Can you work these out from the model? Positions are in its coordinate system, mm. Face numbers are marked on the shaded views. A direction names the side the tool comes from. Coordinates: 2 decimals unless noted, no trailing zeros. Loops run counter-clockwise (first coordinate to the right, second up) from the corner with the lowest first, then second, coordinate; pieces in that order, holes last.
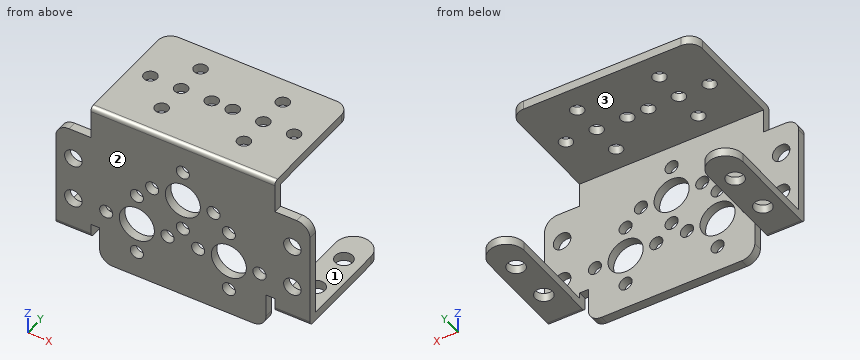
```python
from build123d import *

# Parameters (mm, degrees)
SKETCH1_R               = 2
SKETCH1_R_2             = 4
SKETCH1_R_3             = 1.5
BOSS_EXTRUDE1_DEPTH     = 27
SKETCH3_W               = 28.5
SKETCH3_H               = 26.527175283
SKETCH3_W_2             = 6.268481117
CUT_EXTRUDE1_DEPTH      = 30
CUT_EXTRUDE1_DEPTH_BACK = 30
SKETCH4_R               = 2
SKETCH4_R_2             = 1.5
CUT_EXTRUDE2_DEPTH      = 38.5
SKETCH5_W               = 38
SKETCH5_H               = 27.064125823
CUT_EXTRUDE3_DEPTH      = 27
FILLET1_R               = 3
FILLET2_R               = 1


with BuildPart() as part:
    # Sketch1 → Boss-Extrude1 (new body)
    with BuildSketch(Plane(origin=(0, 0, 0), x_dir=(1, 0, 0), z_dir=(0, 1, 0))):
        with BuildLine():
            Line((21, 0), (-21, 0))
            Line((-21, 0), (-21, 7.5))
            Line((-21, 7.5), (-26, 7.5))
            ThreePointArc((-26, 7.5), (-28.121320344, 8.378679656), (-29, 10.5))
            Line((-29, 10.5), (-29, 32.5))
            Line((-29, 32.5), (-21, 32.5))
            Line((-21, 32.5), (-21, 29.209337349))
            Line((-21, 29.209337349), (-19, 29.209337349))
            Line((-19, 29.209337349), (-19, 34.5))
            ThreePointArc((-19, 34.5), (-18.121320344, 36.621320344), (-16, 37.5))
            Line((-16, 37.5), (16, 37.5))
            ThreePointArc((16, 37.5), (18.121320344, 36.621320344), (19, 34.5))
            Line((19, 34.5), (19, 29.209337349))
            Line((19, 29.209337349), (21, 29.209337349))
            Line((21, 29.209337349), (21, 32.5))
            Line((21, 32.5), (29, 32.5))
            Line((29, 32.5), (29, 10.5))
            ThreePointArc((29, 10.5), (28.121320344, 8.378679656), (26, 7.5))
            Line((26, 7.5), (21, 7.5))
            Line((21, 7.5), (21, 0))
        make_face()
        with Locations((-25, 24.5)):
            Circle(SKETCH1_R, mode=Mode.SUBTRACT)
        with Locations((-25, 14.5)):
            Circle(SKETCH1_R, mode=Mode.SUBTRACT)
        with Locations((25, 14.5)):
            Circle(SKETCH1_R, mode=Mode.SUBTRACT)
        with Locations((25, 24.5)):
            Circle(SKETCH1_R, mode=Mode.SUBTRACT)
        with Locations((0, 14)):
            Circle(SKETCH1_R_2, mode=Mode.SUBTRACT)
        with Locations((0, 21)):
            Circle(SKETCH1_R_3, mode=Mode.SUBTRACT)
        with Locations((7, 14)):
            Circle(SKETCH1_R_3, mode=Mode.SUBTRACT)
        with Locations((0, 7)):
            Circle(SKETCH1_R_3, mode=Mode.SUBTRACT)
        with Locations((-7, 14)):
            Circle(SKETCH1_R_3, mode=Mode.SUBTRACT)
        with Locations((10.5, 24.5)):
            Circle(SKETCH1_R_2, mode=Mode.SUBTRACT)
        with Locations((10.5, 31.5)):
            Circle(SKETCH1_R_3, mode=Mode.SUBTRACT)
        with Locations((-10.5, 24.5)):
            Circle(SKETCH1_R_2, mode=Mode.SUBTRACT)
        with Locations((-10.5, 31.5)):
            Circle(SKETCH1_R_3, mode=Mode.SUBTRACT)
        with Locations((3.5, 24.5)):
            Circle(SKETCH1_R_3, mode=Mode.SUBTRACT)
        with Locations((10.5, 17.5)):
            Circle(SKETCH1_R_3, mode=Mode.SUBTRACT)
        with Locations((17.5, 24.5)):
            Circle(SKETCH1_R_3, mode=Mode.SUBTRACT)
        with Locations((-3.5, 24.5)):
            Circle(SKETCH1_R_3, mode=Mode.SUBTRACT)
        with Locations((-10.5, 17.5)):
            Circle(SKETCH1_R_3, mode=Mode.SUBTRACT)
        with Locations((-17.5, 24.5)):
            Circle(SKETCH1_R_3, mode=Mode.SUBTRACT)
    extrude(amount=BOSS_EXTRUDE1_DEPTH)

    # Sketch3 → Cut-Extrude1 (cut, two sides)
    with BuildSketch(Plane(origin=(0, 0, 0), x_dir=(0, 0, -1), z_dir=(1, 0, 0))) as cut_extrude1_sk:
        with Locations((16.25, 15.263587642)):
            Rectangle(SKETCH3_W, SKETCH3_H)
        with Locations((35.691254192, 15.263587642)):
            Rectangle(SKETCH3_W_2, SKETCH3_H)
    extrude(amount=CUT_EXTRUDE1_DEPTH, mode=Mode.SUBTRACT)
    extrude(cut_extrude1_sk.sketch, amount=-CUT_EXTRUDE1_DEPTH_BACK, mode=Mode.SUBTRACT)

    # Sketch4 → Cut-Extrude2 (cut, through all)
    with BuildSketch(Plane.XY):
        with Locations((-25, 18.573417332)):
            Circle(SKETCH4_R)
        with Locations((-25, 8.573417332)):
            Circle(SKETCH4_R)
        with Locations((-9.391233077, 21.187393838)):
            Circle(SKETCH4_R_2)
        with Locations((-2.391233077, 14.187393838)):
            Circle(SKETCH4_R_2)
        with Locations((-9.391233077, 7.187393838)):
            Circle(SKETCH4_R_2)
        with Locations((-16.391233077, 14.187393838)):
            Circle(SKETCH4_R_2)
        with Locations((2.391233077, 14.187393838)):
            Circle(SKETCH4_R_2)
        with Locations((16.391233077, 14.187393838)):
            Circle(SKETCH4_R_2)
        with Locations((9.391233077, 7.187393838)):
            Circle(SKETCH4_R_2)
        with Locations((9.391233077, 21.187393838)):
            Circle(SKETCH4_R_2)
        with Locations((25, 8.573417332)):
            Circle(SKETCH4_R)
        with Locations((25, 18.573417332)):
            Circle(SKETCH4_R)
        with Locations((-9.391233077, 14.187393838)):
            Circle(SKETCH4_R_2)
        with Locations((9.391233077, 14.187393838)):
            Circle(SKETCH4_R_2)
        with BuildLine():
            Line((-29, 22), (-29, 28.587976658))
            Line((-29, 28.587976658), (-21, 28.587976658))
            Line((-21, 28.587976658), (-21, 22))
            ThreePointArc((-21, 22), (-25, 26), (-29, 22))
        make_face()
        with BuildLine():
            Line((21, 28.587976658), (21, 22))
            ThreePointArc((21, 22), (25, 26), (29, 22))
            Line((29, 22), (29, 28.587976658))
            Line((29, 28.587976658), (21, 28.587976658))
        make_face()
    extrude(amount=-CUT_EXTRUDE2_DEPTH, mode=Mode.SUBTRACT)

    # Sketch5 → Cut-Extrude3 (cut)
    with BuildSketch(Plane(origin=(0, 0, -32.557013634), x_dir=(-1, 0, 0), z_dir=(0, 0, -1))):
        with Locations((0, 15.532062912)):
            Rectangle(SKETCH5_W, SKETCH5_H)
    extrude(amount=-CUT_EXTRUDE3_DEPTH, mode=Mode.SUBTRACT)

    # Fillet1
    fillet1_edges = [part.edges().sort_by_distance(p)[0] for p in [
        (21, 27, -1),
        (-21, 27, -1),
    ]]
    fillet(fillet1_edges, radius=FILLET1_R)

    # Fillet2
    fillet2_edges = [part.edges().sort_by_distance(p)[0] for p in [
        (-25, 0, -32.5),
        (25, 0, -32.5),
        (0, 0, 0),
    ]]
    fillet(fillet2_edges, radius=FILLET2_R)


solid = part.part
```
Item 1: I need wall thicknesses on line 1 along Y through (x, z) = (-25, -31.15); line 2 along Y through (x, z) = (-25, -31.9); line 3 along X through (y, z) = (1.5, -14.5). Which ranges of each line are inside material? Lowest first, please.
Results are:
line 1: y = 0 to 6.57, 10.57 to 16.57, 20.57 to 26
line 2: y = 0.08 to 6.57, 10.57 to 16.57, 20.57 to 26
line 3: x = -29 to -27, -23 to -8.41, -5.59 to -3.97, 3.97 to 5.59, 8.41 to 23, 27 to 29
Item 2: Suppose I cut it at C-C, the plane z = -4.5. Please give me the cut outline in (x, y), plus the area to 3 significant figures.
Results are:
outline: (-21, 0) - (21, 0) - (21, 2) - (-21, 2) - close
area: 84.0 mm2
Item 3: Suppose I cut it at A-A, the plane y = 5. Please give me the cut outline in (x, z), plus the area to 3 significant figures.
Results are:
outline: (-29, -32.5) - (-21, -32.5) - (-21, -30.5) - (-29, -30.5) - close; (-21, -2) - (21, -2) - (21, 0) - (-21, 0) - close; (21, -32.5) - (29, -32.5) - (29, -30.5) - (21, -30.5) - close
area: 116 mm2
Item 4: I'm going to push flat-ended pins straight in: P1, Ø1, axis at x = 4, z = -12, coming from the +Y side; P2, Ø1.8, axis at x = 3.5, z = -24.5, coming from the +Y side; P3, Ø12.5, axis at x = -0.5, y = 9, coming from the -Z side; P4, Ø10.5, axis at x = 10.5, z = -24.5, coming from the -Y side. Where does each tip first touch, or does it pass through?
Results are:
P1: stops at y = 2
P2: passes through
P3: stops at z = -2
P4: stops at y = 0
Item 5: On a 3-axis mill with a long thin cutter (end or side, diameter ignored), from which of +Z, -Z, +X, -X, +Y, -Y can I reach the whole of each face in a straight line? I mean the marked faces 1, 2 and 3. Say none if no direction works.
Results are:
face 1: +Z, +X, -X, +Y
face 2: +Z, -Z, +X, -X, -Y
face 3: -Z, +X, -X, +Y
Item 6: Suppose I cut it at B-B, the plane y = 17.25. Please give me the cut outline in (x, z), plus the area to 3 significant figures.
Results are:
outline: (-29, -32.5) - (-26.5, -32.5) - (-26.5, -30.5) - (-29, -30.5) - close; (-23.5, -32.5) - (-21, -32.5) - (-21, -30.5) - (-23.5, -30.5) - close; (-21, -2) - (21, -2) - (21, 0) - (-21, 0) - close; (21, -32.5) - (23.5, -32.5) - (23.5, -30.5) - (21, -30.5) - close; (26.5, -32.5) - (29, -32.5) - (29, -30.5) - (26.5, -30.5) - close
area: 104 mm2
Item 7: Suppose I cut it at D-D, the plane x = -22. Please give me the cut outline in (y, z), plus the area to 3 significant figures.
Results are:
outline: (0, -31.5) arc R1 ccw to (1, -32.5) - (24.65, -32.5) - (24.65, -30.5) - (2, -30.5) - (2, -7.5) - (0, -7.5) - close
area: 95.1 mm2
